Part model, mm, in its own coordinate system. Face numbers are marked on the shaded views. A direction names the side the tool comes from. Round coordinates to 2 decimals unless told otherwise and drop trailing zeros. Order: outer loops, then holes, each group sorted by start corner. A loop starts at its lowest first (then second) coordinate and runs counter-clockwise, first axis right, second up. Notation, with made-up numbers: M 31.5,37.5 L 66.5,37.5 A18 cw 66.5,66.5 Z; hole C 29,46 d5. An arc over 180 degrees is marked long. One line per question, with ' | ' between items.
from build123d import *

# Parameters (mm, degrees)
SKETCH1_R           = 3.3655
BOSS_EXTRUDE1_DEPTH = 0.7874
SKETCH2_R           = 1.778
BOSS_EXTRUDE2_DEPTH = 9.4742
SKETCH3_R           = 1.336576357
CUT_EXTRUDE1_DEPTH  = 4.3942


with BuildPart() as part:
    # Sketch1 → Boss-Extrude1 (new body)
    with BuildSketch(Plane(origin=(0, 0, 0), x_dir=(1, 0, 0), z_dir=(0, 1, 0))):
        with BuildLine():
            Line((-21.3614, 0), (-21.3614, 1.3335))
            Line((-21.3614, 1.3335), (-15.503317076, 1.3335))
            ThreePointArc((-15.503317076, 1.3335), (-10.252349187, 1.944748659), (-5.282190317, 3.745806542))
            Line((-5.282190317, 3.745806542), (-4.063378909, 4.355050118))
            ThreePointArc((-4.063378909, 4.355050118), (5.9563, 0), (-4.063378909, -4.355050118))
            Line((-4.063378909, -4.355050118), (-5.282190317, -3.745806542))
            ThreePointArc((-5.282190317, -3.745806542), (-10.252349187, -1.944748659), (-15.503317076, -1.3335))
            Line((-15.503317076, -1.3335), (-21.3614, -1.3335))
            Line((-21.3614, -1.3335), (-21.3614, 0))
        make_face()
        with Locations(Location((0, 0, 0), (0, 0, 270))):
            Circle(SKETCH1_R, mode=Mode.SUBTRACT)
    extrude(amount=BOSS_EXTRUDE1_DEPTH)

    # Sketch2 → Boss-Extrude2 (add)
    with BuildSketch(Plane.ZY.offset(21.3614)):
        with Locations((0, 1.176036458)):
            Circle(SKETCH2_R)
    extrude(amount=-BOSS_EXTRUDE2_DEPTH)

    # Sketch3 → Cut-Extrude1 (cut)
    with BuildSketch(Plane.ZY.offset(21.3614)):
        with Locations((0, 1.176036458)):
            Circle(SKETCH3_R)
    extrude(amount=-CUT_EXTRUDE1_DEPTH, mode=Mode.SUBTRACT)


solid = part.part
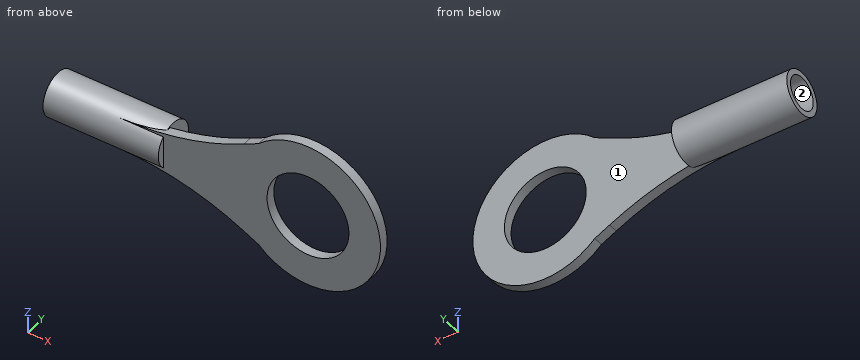
1) Drop flat-ended pins along their axis: pin 1 (0.7 mm diameter, centred on y = -0.5, z = 0.5, fed in from +X); pin 2 (4 mm diameter, centred on x = 0, z = 0, fed in from +Y); pin 3 (3 mm diameter, centred on x = -18.5, z = 2, fed in from +Y); pin 4 (6 mm diameter, centred on x = -4, z = 2, fed in from -Y). Give the stop position or say it passes through.
The answers:
pin 1: stops at x = -11.89 | pin 2: passes through | pin 3: stops at y = 2.88 | pin 4: stops at y = 0
2) Saw through at A-A (z = 0). List the corners of the cut face in (x, y).
The answers:
outline: M -21.36,-0.6 L -11.89,-0.6 L -11.89,0 L -3.37,0 L -3.37,0.79 L -11.89,0.79 L -11.89,2.95 L -21.36,2.95 L -21.36,2.51 L -16.97,2.51 L -16.97,-0.16 L -21.36,-0.16 Z; M 3.37,0 L 5.96,0 L 5.96,0.79 L 3.37,0.79 Z
3) Probe line 1 (X direction, y = 0.5, z = 0); line 2 (Y direction, x = -19.7, z = 0); line 3 (Y direction, x = -7.5, z = 2.25). List the from-to ranges inside material, lowest first. Write a range as [from, to].
The answers:
line 1: x = [-16.97, -3.37], [3.37, 5.96] | line 2: y = [-0.6, -0.16], [2.51, 2.95] | line 3: y = [0, 0.79]
4) Which spindle directions (+Z, -Z, +X, -X, +Y, -Y) get a long thin tool onto all of the face, cutting with end or side? Do the marked faces 1 and 2. Say none if no direction does.
The answers:
face 1: +Z, -Z, +X, +Y | face 2: -X
5) Saw through at C-C (y = 2.2). List the corners of the cut face in (x, z), plus the area to 3 significant figures.
The answers:
outline: M -21.36,-1.45 L -11.89,-1.45 L -11.89,1.45 L -21.36,1.45 L -21.36,0.86 L -16.97,0.86 L -16.97,-0.86 L -21.36,-0.86 Z | area: 20.0 mm²
6) Saw through at B-B (x = -2.75). List the corners of the cut face in (y, z), plus the area to 3 significant figures.
The answers:
outline: M 0,-5.28 L 0.79,-5.28 L 0.79,-1.94 L 0,-1.94 Z; M 0,1.94 L 0.79,1.94 L 0.79,5.28 L 0,5.28 Z | area: 5.27 mm²
